Build history of the part. All positions in model axes, mm. Face numbers are marked on the shaded views. Give positions to 0.01 mm unless a question says otherwise; leave off trailing zeros. Write each loop counter-clockwise with the first axis right and the second up, starting at its lowest first coordinate (ties: lowest second). Pieces come first, ordered by that corner, then holes. Notation, with made-up numbers: (-24.75, 51) - (26.25, 51) arc R24 ccw to (26.25, 73) - close; hole circle Ø2 at (10.5, -20.75). An arc over 180 degrees is marked (long way). Use one line per item in the form item = value. Start each with the question number.
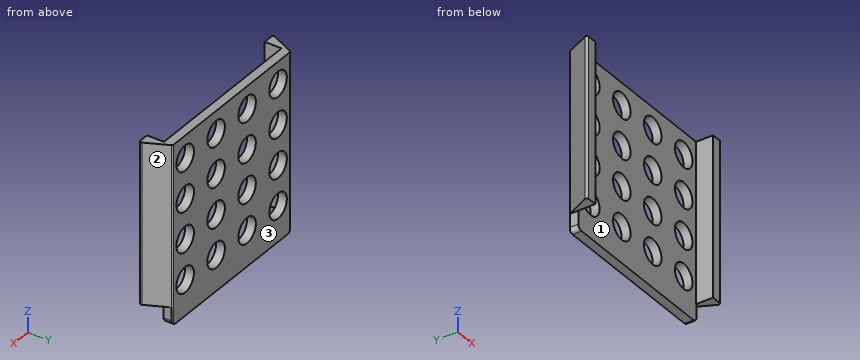
Autodesk Inventor part; units mm, degrees
ref_plane "YZ Plane" through (0, 0, 0) normal (1, 0, 0) x (0, 1, 0)
ref_plane "XZ Plane" through (0, 0, 0) normal (0, 1, 0) x (-1, 0, 0)
ref_plane "XY Plane" through (0, 0, 0) normal (0, 0, 1) x (1, 0, 0)
sketch "Sketch1" plane through (0, 0, 0) normal (0, 0, 1) x (1, 0, 0)
  line L0 (0, 0) -> (19, 0)
  line L1 (19, 0) -> (20.4, 0)
  line L2 (0, 0) -> (-1.4, 0)
  line L3 (0, 0) -> (0, 1.9)
  line L4 (-1.4, 0) -> (0, 2.9)
  line L5 (19, 0) -> (19, 1.9)
  line L6 (19, 2.9) -> (20.4, 0)
  line L7 (0, 2.9) -> (19, 2.9)
  line L8 (0, 1.9) -> (19, 1.9)
  dimension "d0" = 19
  dimension "d1" = 1.4
  dimension "d2" = 1.4
  dimension "d3" = 2.9
  dimension "d4" = 2.9
  dimension "d5" = 1
extrude "Extrusion1" add sketch "Sketch1" along normal blind 20 contours L2 L4 L7 L6 L1 L5 L8 L3
fillet "Fillet1" radius 0.2 4 edges at (0, 2.9, 10) (19, 2.9, 10) (20.4, 0, 10) (-1.4, 0, 10)
sketch "Sketch2" plane through (0, 1.9, 0) normal (0, -1, 0) x (1, 0, 0)
  line L0 (-1.2814, 0) -> (-1.2814, 20)
  line L1 (0, 0) -> (0, 20)
  line L2 (-1.2814, 0) -> (0, 0)
  line L3 (0, 0) -> (0, 2)
  line L4 (0, 2) -> (-1.2814, 2)
  line L5 (-1.2814, 2) -> (-1.2814, 0)
  line L6 (19, 0) -> (19, 20)
  line L7 (20.2814, 0) -> (20.2814, 20)
  line L8 (19, 0) -> (20.2814, 0)
  line L9 (20.2814, 0) -> (20.2814, 2)
  line L10 (20.2814, 2) -> (19, 2)
  line L11 (19, 2) -> (19, 0)
  dimension "d9" = 2
  dimension "d10" = 2
extrude "Extrusion2" cut sketch "Sketch2" along normal blind 20
sketch "Sketch3" plane through (0.1255, 2.9, 0) normal (0, 1, 0) x (1, 0, 0)
  line L0 (-0.1255, -2) -> (-0.6083, -2)
  line L1 (18.7489, 0) -> (18.7489, -20)
  line L2 (-0.1255, -2) -> (18.7489, -2)
  line L3 (18.7489, -2) -> (18.7489, -20)
  line L4 (18.7489, -20) -> (-0.1255, -20)
  line L5 (-0.1255, -20) -> (-0.1255, -2)
  line L6 (-0.1255, -2) -> (-0.1255, -20)
  line L7 (-0.1255, -2) -> (1.8745, -2)
  line L8 (1.8745, -2) -> (1.8745, -4)
  line L9 (0.8745, -5) -> (2.8745, -5)
  line L10 (2.8745, -5) -> (2.8745, -3)
  line L11 (2.8745, -3) -> (0.8745, -3)
  line L12 (0.8745, -3) -> (0.8745, -5)
  line L13 (0.8745, -5) -> (2.8745, -3) construction
  line L14 (2.8745, -5) -> (0.8745, -3) construction
  line L15 (7.8745, -3) -> (5.8745, -3)
  line L16 (5.8745, -3) -> (5.8745, -5)
  line L17 (7.8745, -5) -> (7.8745, -3)
  line L18 (5.8745, -5) -> (7.8745, -5)
  line L19 (12.8745, -3) -> (10.8745, -3)
  line L20 (10.8745, -3) -> (10.8745, -5)
  line L21 (12.8745, -5) -> (12.8745, -3)
  line L22 (10.8745, -5) -> (12.8745, -5)
  line L23 (17.8745, -3) -> (15.8745, -3)
  line L24 (15.8745, -3) -> (15.8745, -5)
  line L25 (17.8745, -5) -> (17.8745, -3)
  line L26 (15.8745, -5) -> (17.8745, -5)
  line L27 (2.8745, -7.5) -> (0.8745, -7.5)
  line L28 (0.8745, -7.5) -> (0.8745, -9.5)
  line L29 (2.8745, -9.5) -> (2.8745, -7.5)
  line L30 (0.8745, -9.5) -> (2.8745, -9.5)
  line L31 (7.8745, -7.5) -> (5.8745, -7.5)
  line L32 (5.8745, -7.5) -> (5.8745, -9.5)
  line L33 (7.8745, -9.5) -> (7.8745, -7.5)
  line L34 (5.8745, -9.5) -> (7.8745, -9.5)
  line L35 (12.8745, -7.5) -> (10.8745, -7.5)
  line L36 (10.8745, -7.5) -> (10.8745, -9.5)
  line L37 (12.8745, -9.5) -> (12.8745, -7.5)
  line L38 (10.8745, -9.5) -> (12.8745, -9.5)
  line L39 (17.8745, -7.5) -> (15.8745, -7.5)
  line L40 (15.8745, -7.5) -> (15.8745, -9.5)
  line L41 (17.8745, -9.5) -> (17.8745, -7.5)
  line L42 (15.8745, -9.5) -> (17.8745, -9.5)
  line L43 (2.8745, -12) -> (0.8745, -12)
  line L44 (0.8745, -12) -> (0.8745, -14)
  line L45 (2.8745, -14) -> (2.8745, -12)
  line L46 (0.8745, -14) -> (2.8745, -14)
  line L47 (7.8745, -12) -> (5.8745, -12)
  line L48 (5.8745, -12) -> (5.8745, -14)
  line L49 (7.8745, -14) -> (7.8745, -12)
  line L50 (5.8745, -14) -> (7.8745, -14)
  line L51 (12.8745, -12) -> (10.8745, -12)
  line L52 (10.8745, -12) -> (10.8745, -14)
  line L53 (12.8745, -14) -> (12.8745, -12)
  line L54 (10.8745, -14) -> (12.8745, -14)
  line L55 (17.8745, -12) -> (15.8745, -12)
  line L56 (15.8745, -12) -> (15.8745, -14)
  line L57 (17.8745, -14) -> (17.8745, -12)
  line L58 (15.8745, -14) -> (17.8745, -14)
  line L59 (2.8745, -16.5) -> (0.8745, -16.5)
  line L60 (0.8745, -16.5) -> (0.8745, -18.5)
  line L61 (2.8745, -18.5) -> (2.8745, -16.5)
  line L62 (0.8745, -18.5) -> (2.8745, -18.5)
  line L63 (7.8745, -16.5) -> (5.8745, -16.5)
  line L64 (5.8745, -16.5) -> (5.8745, -18.5)
  line L65 (7.8745, -18.5) -> (7.8745, -16.5)
  line L66 (5.8745, -18.5) -> (7.8745, -18.5)
  line L67 (12.8745, -16.5) -> (10.8745, -16.5)
  line L68 (10.8745, -16.5) -> (10.8745, -18.5)
  line L69 (12.8745, -18.5) -> (12.8745, -16.5)
  line L70 (10.8745, -18.5) -> (12.8745, -18.5)
  line L71 (17.8745, -16.5) -> (15.8745, -16.5)
  line L72 (15.8745, -16.5) -> (15.8745, -18.5)
  line L73 (17.8745, -18.5) -> (17.8745, -16.5)
  line L74 (15.8745, -18.5) -> (17.8745, -18.5)
  circle A0 centre (1.8745, -4) radius 1.4142
  circle A1 centre (6.8745, -4) radius 1.4142
  circle A2 centre (11.8745, -4) radius 1.4142
  circle A3 centre (16.8745, -4) radius 1.4142
  circle A4 centre (1.8745, -8.5) radius 1.4142
  circle A5 centre (6.8745, -8.5) radius 1.4142
  circle A6 centre (11.8745, -8.5) radius 1.4142
  circle A7 centre (16.8745, -8.5) radius 1.4142
  circle A8 centre (1.8745, -13) radius 1.4142
  circle A9 centre (6.8745, -13) radius 1.4142
  circle A10 centre (11.8745, -13) radius 1.4142
  circle A11 centre (16.8745, -13) radius 1.4142
  circle A12 centre (1.8745, -17.5) radius 1.4142
  circle A13 centre (6.8745, -17.5) radius 1.4142
  circle A14 centre (11.8745, -17.5) radius 1.4142
  circle A15 centre (16.8745, -17.5) radius 1.4142
  point P0 (-0.1255, 0)
  dimension "d13" = 2
  dimension "d14" = 2
  dimension "d15" = 2
  dimension "d16" = 2
  dimension "d19" = 5
  dimension "d22" = 4.5
  dimension "d32" = 5
  dimension "d35" = 4.5
extrude "Extrusion3" cut sketch "Sketch3" against normal through all contours A0 L11 L8 | L8 L11 A0 | L11 L10 L9 L12 | A0 L10 | L12 A0 | A0 L9 | L17 L18 L16 L15 | A1 L17 | L15 A1 | L16 A1 | A1 L18 | L21 L22 L20 L19 | A2 L21 | L19 A2 | L20 A2 | A2 L22 | L25 L26 L24 L23 | A3 L25 | L23 A3 | L24 A3 | A3 L26 | L29 L30 L28 L27 | A4 L29 | L27 A4 | L28 A4 | A4 L30 | L33 L34 L32 L31 | A5 L33 | L31 A5 | L32 A5 | A5 L34 | L37 L38 L36 L35 | A6 L37 | L35 A6 | L36 A6 | A6 L38 | L41 L42 L40 L39 | A7 L41 | L39 A7 | L40 A7 | A7 L42 | L45 L46 L44 L43 | A8 L45 | L43 A8 | L44 A8 | A8 L46 | L49 L50 L48 L47 | A9 L49 | L47 A9 | L48 A9 | A9 L50 | L53 L54 L52 L51 | A10 L53 | L51 A10 | L52 A10 | A10 L54 | L57 L58 L56 L55 | A11 L57 | L55 A11 | L56 A11 | A11 L58 | L61 L62 L60 L59 | A12 L61 | L59 A12 | L60 A12 | A12 L62 | L65 L66 L64 L63 | A13 L65 | L63 A13 | L64 A13 | A13 L66 | L69 L70 L68 L67 | A14 L69 | L67 A14 | L68 A14 | A14 L70 | L73 L74 L72 L71 | A15 L73 | L71 A15 | L72 A15 | A15 L74
sketch "Sketch4" plane through (-0.4828, 1.9, 0) normal (0, -1, 0) x (1, 0, 0)
  line L0 (0, 0) -> (0, 2)
  line L1 (0, 2) -> (0.4828, 2)
  line L2 (0.4828, 2) -> (0.4828, 0)
  line L3 (0.4828, 0) -> (0, 0)
  line L4 (0, 0) -> (0, 2)
  line L5 (19.9655, 2) -> (19.9655, 0)
  line L6 (19.9655, 0) -> (19.5373, 0)
  line L7 (19.9655, 2) -> (19.5373, 2)
  line L8 (19.5373, 2) -> (19.5373, 0)
  line L9 (19.5373, 0) -> (19.9655, 0)
  line L10 (19.9655, 0) -> (19.9655, 2)
extrude "Extrusion4" cut sketch "Sketch4" against normal blind 20
fillet "Fillet2" radius 0.5 2 edges at (19.0546, 2.3435, 0) (0, 2.3778, 0)
properties part number "flange2_grip_support"
(1) Pin check, flat tips, straight feed: pin 1 Ø4.5 at (x, z) = (12, 17.5) entering from -Y; pin 2 Ø0.5 at (y, z) = (2.5, 1.5) entering from -X; pin 3 Ø1.4 at (x, y) = (-1, 1) entering from -Z. Stop position of each tip, or through.
(2) Wall check: line 1 (Z direction, x = 2, y = 2.55); line 2 (X direction, y = 0.25, z = 12.5); line 3 (X direction, y = 2.3, z = 13). Give the ranges that are in metal, low to high. Write a range as from..to.
(3) Cut at A-A, the plane z = 17.5. Give the cut face in (x, y).
(4) Cut at C-C, the plane y = 1.5. Give the cut face in (x, z).
(5) Cut at D-D, the plane z = 13.5. Give the cut face in (x, y).
(6) Cut at B-B, the plane x = 3. Give the cut face in (y, z).
(7) Two-plate mould, pull along X, no slides. Class the marked faces 1, 2 and 3: +X half, -X half, draft (parallel to the pull), parting line (faces both ways), or undercut.
Solution:
q1.pin_1 = 1.9
q1.pin_2 = 0
q1.pin_3 = 2
q2.line_1 = 0..2.59, 5.41..7.09, 9.91..11.59, 14.41..16.09, 18.91..20
q2.line_2 = -1.28..0, 19..20.28
q2.line_3 = -0.29..0.59, 3.41..5.59, 8.41..10.59, 13.41..15.59, 18.41..19.29
q3.outline = (-1.26, 0.29) arc R0.2 ccw to (-1.08, 0) - (0, 0) - (0, 1.9) - (0.59, 1.9) - (0.59, 2.9) - (0.13, 2.9) arc R0.2 ccw to (-0.05, 2.79) - close; (3.41, 1.9) - (5.59, 1.9) - (5.59, 2.9) - (3.41, 2.9) - close; (8.41, 1.9) - (10.59, 1.9) - (10.59, 2.9) - (8.41, 2.9) - close; (13.41, 1.9) - (15.59, 1.9) - (15.59, 2.9) - (13.41, 2.9) - close; (18.41, 1.9) - (19, 1.9) - (19, 0) - (20.08, 0) arc R0.2 ccw to (20.26, 0.29) - (19.05, 2.79) arc R0.2 ccw to (18.87, 2.9) - (18.41, 2.9) - close
q4.outline = (-0.68, 2) - (0, 2) - (0, 20) - (-0.68, 20) - close; (19, 2) - (19.68, 2) - (19.68, 20) - (19, 20) - close
q5.outline = (-1.26, 0.29) arc R0.2 ccw to (-1.08, 0) - (0, 0) - (0, 1.9) - (0.68, 1.9) - (0.68, 2.9) - (0.13, 2.9) arc R0.2 ccw to (-0.05, 2.79) - close; (3.32, 1.9) - (5.68, 1.9) - (5.68, 2.9) - (3.32, 2.9) - close; (8.32, 1.9) - (10.68, 1.9) - (10.68, 2.9) - (8.32, 2.9) - close; (13.32, 1.9) - (15.68, 1.9) - (15.68, 2.9) - (13.32, 2.9) - close; (18.32, 1.9) - (19, 1.9) - (19, 0) - (20.08, 0) arc R0.2 ccw to (20.26, 0.29) - (19.05, 2.79) arc R0.2 ccw to (18.87, 2.9) - (18.32, 2.9) - close
q6.outline = (1.9, 0) - (2.9, 0) - (2.9, 3) - (1.9, 3) - close; (1.9, 5) - (2.9, 5) - (2.9, 7.5) - (1.9, 7.5) - close; (1.9, 9.5) - (2.9, 9.5) - (2.9, 12) - (1.9, 12) - close; (1.9, 14) - (2.9, 14) - (2.9, 16.5) - (1.9, 16.5) - close; (1.9, 18.5) - (2.9, 18.5) - (2.9, 20) - (1.9, 20) - close
q7.face_1 = undercut
q7.face_2 = +X half
q7.face_3 = draft
